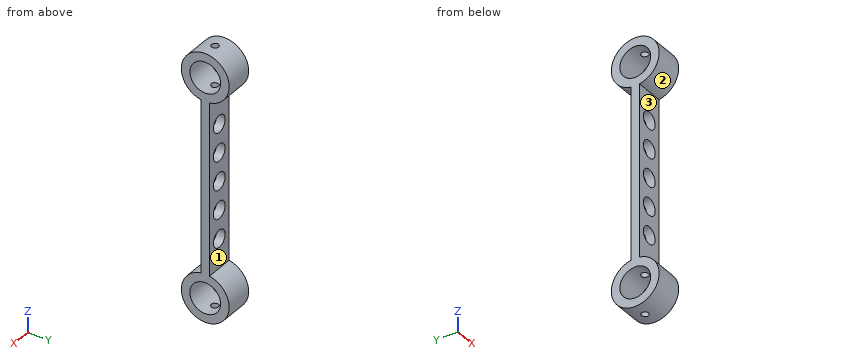
Autodesk Inventor part; units mm, degrees
ref_plane "작업 평면1" through (0, 0, -8.4) normal (0, 0, 1) x (1, 0, 0)
ref_plane "작업 평면4" through (0, 0, -68.4) normal (0, 0, 1) x (1, 0, 0)
ref_plane "YZ Plane" through (0, 0, 0) normal (1, 0, 0) x (0, 1, 0)
sketch "스케치1" plane through (0, 0, 0) normal (1, 0, 0) x (0, 1, 0)
  circle A0 centre (0, 0) radius 5.4
  circle A1 centre (0, 0) radius 8.4
  line L0 (34.8065, -38.4) -> (-35.3174, -38.4) construction
  circle A2 centre (0, -76.8) radius 5.4
  circle A3 centre (0, -76.8) radius 8.4
  dimension "d0" = 10.8
  dimension "d1" = 16.8
  dimension "d4" = 38.4
extrude "돌출1" add sketch "스케치1" along normal blind 10
ref_plane "작업 평면1" through (0, 0, -8.4) normal (0, 0, 1) x (1, 0, 0)
sketch "스케치2" plane through (0, 0, -8.4) normal (0, 0, 1) x (1, 0, 0)
  line L0 (10, -8.4) -> (10, 8.4)
  line L1 (0, -8.4) -> (0, 8.4)
  line L2 (0, 8.4) -> (10, 8.4)
  line L3 (0, -8.4) -> (10, -8.4)
  line L4 (0, -8.4) -> (0, 8.4)
  line L5 (10, -1.5) -> (0, -1.5)
  line L6 (0, -1.5) -> (0, 1.5)
  line L7 (0, 1.5) -> (10, 1.5)
  line L8 (10, 1.5) -> (10, -1.5)
  line L9 (10, -1.5) -> (0, 1.5) construction
  line L10 (0, -1.5) -> (10, 1.5) construction
  point P0 (0, 0)
  point P1 (5, 0)
  point P2 (0, -1.5)
  dimension "d6" = 8.4
  dimension "d7" = 3
  dimension "d12" = 10
extrude "돌출2" add sketch "스케치2" along normal blind 3 contours L5 L1 L7 L0
extrude "돌출3" add sketch "스케치2" against normal blind 63 contours L5 L1 L7 L0
sketch "스케치4" plane through (0, 1.5, -8.265) normal (0, 1, 0) x (1, 0, 0)
  line L0 (0, 0) -> (0, 60.27)
  line L1 (10, 0) -> (0, 0)
  line L2 (0, 60.27) -> (10, 60.27)
  line L3 (10, 0) -> (10, 60.27)
  line L4 (0, 60.27) -> (0, 0)
  line L5 (5, -0.4) -> (5, 39.3864) construction
  circle A0 centre (5, 30) radius 3
  circle A1 centre (5, 40) radius 3
  circle A2 centre (5, 50) radius 3
  circle A3 centre (5, 20) radius 3
  circle A4 centre (5, 10) radius 3
  point P0 (0, -8.265)
  dimension "d22" = 6
  dimension "d23" = 30
  dimension "d26" = 10
  dimension "d33" = 10
ref_plane "작업 평면3" through (0, 0, -8.4) normal (0, 0, 1) x (1, 0, 0)
ref_plane "작업 평면4" through (0, 0, -68.4) normal (0, 0, 1) x (1, 0, 0)
extrude "돌출4" cut sketch "스케치4" against normal blind 10 contours A0 | A1 | A2 | A3 | A4
ref_plane "작업 평면6" through (0, 0, -85.2) normal (0, 0, 1) x (1, 0, 0)
ref_plane "작업 평면5" through (0, 0, 8.4) normal (0, 0, 1) x (1, 0, 0)
sketch "스케치5" plane through (0, 0, 8.4) normal (0, 0, 1) x (1, 0, 0)
  line L0 (10, 1.5) -> (0, 1.5)
  line L1 (0, 1.5) -> (0, -1.5)
  line L2 (0, -1.5) -> (10, -1.5)
  line L3 (10, 1.5) -> (10, -1.5)
  line L4 (0, 8.4) -> (10, 8.4)
  line L5 (0, -8.4) -> (0, 8.4)
  line L6 (10, -8.4) -> (10, 8.4)
  line L7 (0, -8.4) -> (10, -8.4)
  circle A0 centre (5, 0) radius 1.25
  point P0 (0, 0)
  dimension "d40" = 2.5
  dimension "d41" = 5
  dimension "d42" = 8.4
sketch "스케치6" plane through (0, 0, -85.2) normal (0, 0, 1) x (1, 0, 0)
  circle A0 centre (5, 0) radius 1.25
  line L0 (0, 8.4) -> (10, 8.4)
  line L1 (10, -8.4) -> (10, 8.4)
  line L2 (10, -1.5) -> (0, -1.5)
  line L3 (0, -1.5) -> (0, 1.5)
  line L4 (0, 1.5) -> (10, 1.5)
  line L5 (10, -1.5) -> (10, 1.5)
  line L6 (2, 1.5) -> (2, -1.5)
  line L7 (0, -8.4) -> (0, 8.4)
  point P0 (0, 0)
  dimension "d46" = 2.5
  dimension "d47" = 8.4
  dimension "d48" = 5
extrude "돌출5" cut sketch "스케치6" along normal blind 17 contours A0
extrude "돌출6" cut sketch "스케치5" against normal blind 17 contours A0
properties part number "link"
Could you check a few things on this model? Use its own coordinates, in mm. Face numbers are marked on the shaded views. A direction names the side the tool comes from. Round coordinates to 2 decimals unless told otherwise and drop trailing zeros. Order: outer loops, then holes, each group sorted by start corner. A loop starts at its lowest first (then second) coordinate and runs counter-clockwise, first axis right, second up. Notation, with made-up numbers: M 64,-13.75 L 77,-13.75 A17 ccw 77,9.25 Z; hole C 42.25,72.25 d1. An arc over 180 degrees is marked long. One line per item, written item: value.
(1) Which directions (+Z, -Z, +X, -X, +Y, -Y) give clear straight access to the entire face, cutting with the end or side of a thin tool? Please do the marked faces 1, 2 and 3.
Ans:
face 1: +X, -X, +Y
face 2: +X, -X
face 3: +X, -X, -Y
(2) Imagine slicing it at A-A (z = -76.8). Write out the boundary of the cut face in (x, y), and give its area (3 significant figures).
Ans:
outline: M 0,-8.4 L 10,-8.4 L 10,-5.4 L 0,-5.4 Z; M 0,5.4 L 10,5.4 L 10,8.4 L 0,8.4 Z
area: 60.0 mm^2
(3) I need wall thicknesses on line 1 along Z through (x, y) = (5, 0.55) (3 decimals); line 2 along Z through (x, y) = (7, -3.5); line 3 along Z through (x, y) = (7.75, 2). Which ranges of each line are inside material? Lowest first, please. Write a range as from..to.
Ans:
line 1: z = -68.2..-61.265, -55.265..-51.265, -45.265..-41.265, -35.265..-31.265, -25.265..-21.265, -15.265..-8.6
line 2: z = -84.44..-80.91, -72.69..-69.16, -7.64..-4.11, 4.11..7.64
line 3: z = -84.96..-81.82, -71.78..-68.64, -8.16..-5.02, 5.02..8.16
(4) Imagine slicing it at C-C (y = -7). Write out the boundary of the cut face in (x, z), and give its area (3 significant figures).
Ans:
outline: M 0,-81.44 L 10,-81.44 L 10,-72.16 L 0,-72.16 Z; M 0,-4.64 L 10,-4.64 L 10,4.64 L 0,4.64 Z
area: 186 mm^2
(5) I'm going to push flat-ended pins straight in: P1, Ø3, axis at x = 8, y = -5.5, coming from the +Z side; P2, Ø1.5, axis at x = 5, y = 0, coming from the -Z side; P3, Ø1.5, axis at x = 8.5, y = 3.5, coming from the -Z side. Where does each tip first touch, or does it pass through?
Ans:
P1: stops at z = 7.39
P2: stops at z = -68.2
P3: stops at z = -84.74
(6) Imagine slicing it at B-B (y = 0). Count the separate pieces of the cut face and the enclosed holes in it, and give its area (3 significant figures).
Ans:
separate pieces: 5
enclosed holes: 5
area: 548 mm^2
